Verification items for the finished model (mm, model axes). A direction names the side the tool comes from. Coordinates: 2 decimals unless noted, no trailing zeros. Order: outer loops, then holes, each group sorted by start corner. A loop starts at its lowest first (then second) coordinate and runs counter-clockwise, first axis right, second up.
Q1. Cross-section at D-D, the plane z = 38.5. Record the boundary of the cut face in (x, y).
Q2. Cross-section at B-B, the plane z = 26.5. Record the boundary of the cut face in (x, y).
Q3. Cross-section at A-A, the plane x = -47. Record the boundary of the cut face in (y, z).
Q4. Depth check by flat-ended pin: P1, Ø1.9, axis at x = -45, y = -9.5, coming from the -Z side; P2, Ø4.5, axis at y = -6.5, z = 28, coming from the +X side; P3, Ø4, axis at y = -6.5, z = 41.5, coming from the -X side. Enter the tip coordinate at first touch or a pass-through.
Q5. Draft check along Z on faces 1 (the flat face through (0, -4, 35)), 2 (the cylindrical face through (-78, -4, 49)), 3 (the flat face through (-42, -9, 53.303)). Enter one of: pulls with the +Z half, pulls with the -Z half, needs draft (parallel to the pull), parting line crosses it, or undercut.
Q6. Thickness scan on line 1 (X direction, y = -8.5, z = 37.5); line 2 (X direction, y = -4.25, z = 50.5); line 3 (Y direction, x = -47.5, z = 28). Record the ranges inside material, lowest first.
Q7. Set-up check for faces 4 (the flat face through (-42, -8.3, 55)), 5 (the flat face through (-83.274, -3, 40)), 6 (the flat face through (-42, -3, 13.395)): record each of +Z, -Z, +X, -X, +Y, -Y from which the full face is reachable in a straight line by a thin tool's end or side.
Q8. Cross-section at C-C, the plane x = -24. Record the boundary of the cut face in (y, z), and give its area (3 significant figures).
from build123d import *

# Parameters (mm, degrees)
F0_W      = 86
F0_H      = 50
F1_DEPTH  = 1
F2_W      = 26
F2_H      = 50
F3_DEPTH  = 9
F4_W      = 13
F4_H      = 47
F5_DEPTH  = 8
F6_W      = 13
F6_H      = 4.0918802842
F7_DEPTH  = 2
F8_W      = 13
F8_H      = 1.7
F9_DEPTH  = 3
F11_DEPTH = 28
F13_DEPTH = 28
F14_W     = 2
F14_H     = 50
F15_DEPTH = 3
F16_R     = 3
F17_R     = 2.75
F18_DEPTH = 6.5
F19_R     = 2
F20_R     = 3


with BuildPart() as f1:
    # F0 (on Front) → F1 (new body)
    with BuildSketch(Plane.XZ):
        with Locations((-42.2739830759, 34.3034887686)):
            Rectangle(F0_W, F0_H)
    extrude(amount=F1_DEPTH)

    # F2 (on face) → F3 (join)
    with BuildSketch(Plane.XZ.offset(1)):
        with Locations((-42.2739830759, 34.3034887686)):
            Rectangle(F2_W, F2_H)
    extrude(amount=F3_DEPTH)

    # F4 (on face) → F5 (cut)
    with BuildSketch(Plane.XZ.offset(10)):
        with Locations((-42.2739830759, 32.8034887686)):
            Rectangle(F4_W, F4_H)
    extrude(amount=-F5_DEPTH, mode=Mode.SUBTRACT)

    # F6 (on face) → F7 (join)
    with BuildSketch(Plane.XZ.offset(2)):
        with Locations((-42.2739830759, 11.3494289108)):
            Rectangle(F6_W, F6_H)
    extrude(amount=F7_DEPTH)

    # F8 (on face) → F9 (join)
    with BuildSketch(Plane(origin=(0, 0, 56.3034887686), x_dir=(1, 0, 0), z_dir=(0, 0, -1))):
        with Locations((-42.2739830759, 9.15)):
            Rectangle(F8_W, F8_H)
    extrude(amount=F9_DEPTH)

    # F10 (on face) → F11 (join)
    with BuildSketch(Plane(origin=(-55.2739830759, 0, 0), x_dir=(0, -1, 0), z_dir=(-1, 0, 0))):
        Polygon((3, 9.3034887686), (1, 59.3034887686), (1, 9.3034887686), align=None)
    extrude(amount=F11_DEPTH)

    # F12 (on face) → F13 (join)
    with BuildSketch(Plane.YZ.offset(-29.2739830759)):
        Polygon((-1, 9.3034887686), (-1, 59.3034887686), (-3, 9.3034887686), align=None)
    extrude(amount=F13_DEPTH)

    # F14 (on face) → F15 (join)
    with BuildSketch(Plane.XZ.offset(1)):
        with Locations((-0.2739830759, 34.3034887686)):
            Rectangle(F14_W, F14_H)
        with Locations((-84.2739830759, 34.3034887686)):
            Rectangle(F14_W, F14_H)
    extrude(amount=F15_DEPTH)

    # F16
    f16_edges = [f1.edges().sort_by_distance(p)[0] for p in [
        (-85.273983, 0, 34.303489),
        (0.726017, 0, 34.303489),
    ]]
    fillet(f16_edges, radius=F16_R)

    # F17 (on face) → F18 (join)
    with BuildSketch(Plane(origin=(0, -3.3667527464, 0.1346701099), x_dir=(1, 0, 0), z_dir=(0, -0.9992009587, 0.0399680383))):
        with Locations((-9.2739830759, 49.176150782)):
            Circle(F17_R)
        with Locations((-9.2739830759, 19.176150782)):
            Circle(F17_R)
        with Locations((-75.2739830759, 49.176150782)):
            Circle(F17_R)
        with Locations((-75.2739830759, 19.176150782)):
            Circle(F17_R)
    extrude(amount=F18_DEPTH)

    # F19
    f19_edges = [f1.edges().sort_by_distance(p)[0] for p in [
        (-78.023983, -7.896085, 49.531319),
        (-78.023983, -9.095126, 19.555291),
        (-12.023983, -7.896085, 49.531319),
        (-12.023983, -9.095126, 19.555291),
    ]]
    fillet(f19_edges, radius=F19_R)

    # F20
    f20_edges = [f1.edges().sort_by_distance(p)[0] for p in [
        (-29.273983, -5.5, 59.303489),
        (-55.273983, -5.5, 59.303489),
        (-29.273983, -6.5, 9.303489),
        (-55.273983, -6.5, 9.303489),
    ]]
    fillet(f20_edges, radius=F20_R)


solid = f1.part
Check values:
1. outline: (-85.27, -4) - (-83.27, -4) - (-83.27, -1.83) - (-55.27, -1.83) - (-55.27, -10) - (-48.77, -10) - (-48.77, -2) - (-35.77, -2) - (-35.77, -10) - (-29.27, -10) - (-29.27, -1.83) - (-1.27, -1.83) - (-1.27, -4) - (0.73, -4) - (0.73, -3) arc R3 ccw to (-2.27, 0) - (-82.27, 0) arc R3 ccw to (-85.27, -3) - close
2. outline: (-85.27, -4) - (-83.27, -4) - (-83.27, -2.31) - (-55.27, -2.31) - (-55.27, -10) - (-48.77, -10) - (-48.77, -2) - (-35.77, -2) - (-35.77, -10) - (-29.27, -10) - (-29.27, -2.31) - (-1.27, -2.31) - (-1.27, -4) - (0.73, -4) - (0.73, -3) arc R3 ccw to (-2.27, 0) - (-82.27, 0) arc R3 ccw to (-85.27, -3) - close
3. outline: (-10, 53.3) - (-8.3, 53.3) - (-8.3, 56.3) - (-2, 56.3) - (-2, 13.4) - (-4, 13.4) - (-4, 9.3) - (0, 9.3) - (0, 59.3) - (-10, 59.3) - close
4. P1: stops at z = 53.3
4. P2: stops at x = -29.27
4. P3: stops at x = -55.27
5. face 1: needs draft
5. face 2: undercut
5. face 3: pulls with the -Z half
6. line 1: x = -55.27 to -48.77, -35.77 to -29.27
6. line 2: x = -77.79 to -72.76, -55.27 to -48.77, -35.77 to -29.27, -11.79 to -6.76
6. line 3: y = -2 to 0
7. face 4: -Z
7. face 5: +Z, -Y
7. face 6: -Y
8. outline: (-3, 9.3) - (0, 9.3) - (0, 59.3) - (-1, 59.3) - close
8. area: 100 mm2
